Check sheet for the modelled part. Datum: model origin and axes. Units: mm. Round coordinates to 2 decimals unless told otherwise and drop trailing zeros. Loops run counter-clockwise (first coordinate to the right, second up) from the corner with the lowest first, then second, coordinate; pieces in that order, holes last. Notation, with made-up numbers: (-21.75, -31) -> (-8.75, -31) arc R24 ccw to (-8.75, -3) -> close; hole circle Ø2 at (76, 18.25). An arc over 180 degrees is marked (long way). One line per item, written item: value. Start each with the question number.
1. Cross-section at A-A on x = 0. Record the cut outline in (y, z).
2. Material ranges on L1, parallel to X at y = -7, z = 1.45; L2, parallel to Y at x = 6.5, z = 2.85; L3, parallel to Y at x = -5.5, z = 2.55, recorded low to high.
3. Release check for a two-part mould opening along X. For faces 1 (the face through (0, -28, 1)), 2 (the face through (5.18, -23.33, 1.48)), 3 (the face through (-10, -9, 1)) record: +X half, -X half, draft (parallel to the pull), parting line (faces both ways), or undercut.
4. Go/stop test with flat-tipped pins: pin 1 (1.5 mm diameter, centred on x = -1.5, z = 2.5, fed in from +Y); pin 2 (4.5 mm diameter, centred on x = 0, y = 0, fed in from +Z); pin 3 (5 mm diameter, centred on x = -4.5, y = -21.87, fed in from -Z). Record where each tip stops, or that it passes through.
5. Cross-section at D-D on y = 0.5. Record the cut outline in (x, z), then the cut area to 3 significant figures.
6. Cross-section at B-B on y = -17.5. Record the cut outline in (x, z).
7. Cross-section at C-C on z = 1.05. Count the separate pieces of the cut face and the enclosed holes in it, then the cut area to 3 significant figures.
from build123d import *

# Parameters (mm, degrees)
ESQUISSE1_R        = 3.75
ESQUISSE1_R_2      = 1.5
BOSS_EXTRU_1_DEPTH = 3


with BuildPart() as part:
    # Esquisse1 → Boss.-Extru.1 (new body)
    with BuildSketch(Plane.XY):
        with BuildLine():
            Line((-10, -18), (-10, 0))
            ThreePointArc((-10, 0), (0, 10), (10, 0))
            Line((10, 0), (10, -18))
            ThreePointArc((10, -18), (0, -28), (-10, -18))
        make_face()
        Circle(ESQUISSE1_R, mode=Mode.SUBTRACT)
        with Locations((-4.496614477, -21.867219529)):
            Circle(ESQUISSE1_R_2, mode=Mode.SUBTRACT)
        with Locations((0.503385523, -21.867219529)):
            Circle(ESQUISSE1_R_2, mode=Mode.SUBTRACT)
        with Locations((5.503385523, -21.867219529)):
            Circle(ESQUISSE1_R_2, mode=Mode.SUBTRACT)
        with Locations((0.503385523, -16.867219529)):
            Circle(ESQUISSE1_R_2, mode=Mode.SUBTRACT)
        with Locations((5.503385523, -16.867219529)):
            Circle(ESQUISSE1_R_2, mode=Mode.SUBTRACT)
        with Locations((0.503385523, -11.867219529)):
            Circle(ESQUISSE1_R_2, mode=Mode.SUBTRACT)
        with Locations((5.503385523, -11.867219529)):
            Circle(ESQUISSE1_R_2, mode=Mode.SUBTRACT)
        with Locations((0.503385523, -6.867219529)):
            Circle(ESQUISSE1_R_2, mode=Mode.SUBTRACT)
        with Locations((5.503385523, -6.867219529)):
            Circle(ESQUISSE1_R_2, mode=Mode.SUBTRACT)
        with Locations((-4.496614477, -16.867219529)):
            Circle(ESQUISSE1_R_2, mode=Mode.SUBTRACT)
        with Locations((-4.496614477, -11.867219529)):
            Circle(ESQUISSE1_R_2, mode=Mode.SUBTRACT)
        with Locations((-4.496614477, -6.867219529)):
            Circle(ESQUISSE1_R_2, mode=Mode.SUBTRACT)
    extrude(amount=BOSS_EXTRU_1_DEPTH)


solid = part.part
Taken from the geometry:
1. outline: (-28, 0) -> (-23.28, 0) -> (-23.28, 3) -> (-28, 3) -> close; (-20.45, 0) -> (-18.28, 0) -> (-18.28, 3) -> (-20.45, 3) -> close; (-15.45, 0) -> (-13.28, 0) -> (-13.28, 3) -> (-15.45, 3) -> close; (-10.45, 0) -> (-8.28, 0) -> (-8.28, 3) -> (-10.45, 3) -> close; (-5.45, 0) -> (-3.75, 0) -> (-3.75, 3) -> (-5.45, 3) -> close; (3.75, 0) -> (10, 0) -> (10, 3) -> (3.75, 3) -> close
2. L1: x = -10 to -5.99, -3 to -0.99, 2 to 4.01, 7 to 10
2. L2: y = -25.6 to -22.99, -20.75 to -17.99, -15.75 to -12.99, -10.75 to -7.99, -5.75 to 7.6
2. L3: y = -26.35 to -22.98, -20.75 to -17.98, -15.75 to -12.98, -10.75 to -7.98, -5.75 to 8.35
3. face 1: parting line
3. face 2: undercut
3. face 3: -X half
4. pin 1: stops at y = 9.97
4. pin 2: passes through
4. pin 3: stops at z = 0
5. outline: (-9.99, 0) -> (-3.72, 0) -> (-3.72, 3) -> (-9.99, 3) -> close; (3.72, 0) -> (9.99, 0) -> (9.99, 3) -> (3.72, 3) -> close
5. area: 37.6 mm2
6. outline: (-10, 0) -> (-5.86, 0) -> (-5.86, 3) -> (-10, 3) -> close; (-3.14, 0) -> (-0.86, 0) -> (-0.86, 3) -> (-3.14, 3) -> close; (1.86, 0) -> (4.14, 0) -> (4.14, 3) -> (1.86, 3) -> close; (6.86, 0) -> (10, 0) -> (10, 3) -> (6.86, 3) -> close
7. separate pieces: 1
7. enclosed holes: 13
7. area: 545 mm2
